```python
from build123d import *

# Parameters (mm, degrees)
SKETCH1_W               = 1041.4
SKETCH1_H               = 785.8125
BOSS_EXTRUDE1_DEPTH     = 6.35
CUT_EXTRUDE5_DEPTH      = 1305.62851711
F_1_4_CLEARANCE_HOLE1_D = 7.14248
CUT_EXTRUDE6_DEPTH      = 1305.62851711
SKETCH13_W              = 57.15
SKETCH13_H              = 25.4
CUT_EXTRUDE7_DEPTH      = 1305.62851711
FILLET1_R               = 6.35
FILLET1_OF_MIRROR1_R    = 6.35
CUT_EXTRUDE8_DEPTH      = 1305.62851711
LPATTERN1_COUNT         = 5
LPATTERN1_PITCH         = 222.25
CUT_EXTRUDE9_DEPTH      = 1305.62851711
LPATTERN2_COUNT         = 2
LPATTERN2_PITCH         = 457.2
FILLET2_R               = 6.35


with BuildPart() as part:
    # Sketch1 → Boss-Extrude1 (new body)
    with BuildSketch(Plane.XY):
        with Locations((520.7, 392.90625)):
            Rectangle(SKETCH1_W, SKETCH1_H)
    extrude(amount=BOSS_EXTRUDE1_DEPTH)

    # Sketch11 → Cut-Extrude5 (cut, through all)
    with BuildSketch(Plane.XY.offset(6.35)):
        with BuildLine():
            Line((346.3925, 640.207), (346.3925, 705.2945))
            ThreePointArc((346.3925, 705.2945), (343.2175, 708.4695), (346.3925, 711.6445))
            Line((346.3925, 711.6445), (354.0125, 711.6445))
            ThreePointArc((354.0125, 711.6445), (357.1875, 708.4695), (354.0125, 705.2945))
            Line((354.0125, 705.2945), (354.0125, 640.207))
            ThreePointArc((354.0125, 640.207), (357.1875, 637.032), (354.0125, 633.857))
            Line((354.0125, 633.857), (346.3925, 633.857))
            ThreePointArc((346.3925, 633.857), (343.2175, 637.032), (346.3925, 640.207))
        make_face()
        with BuildLine():
            Line((695.0075, 633.857), (687.3875, 633.857))
            ThreePointArc((687.3875, 633.857), (684.2125, 637.032), (687.3875, 640.207))
            Line((687.3875, 640.207), (687.3875, 705.2945))
            ThreePointArc((687.3875, 705.2945), (684.2125, 708.4695), (687.3875, 711.6445))
            Line((687.3875, 711.6445), (695.0075, 711.6445))
            ThreePointArc((695.0075, 711.6445), (698.1825, 708.4695), (695.0075, 705.2945))
            Line((695.0075, 705.2945), (695.0075, 640.207))
            ThreePointArc((695.0075, 640.207), (698.1825, 637.032), (695.0075, 633.857))
        make_face()
    extrude(amount=-CUT_EXTRUDE5_DEPTH, mode=Mode.SUBTRACT)

    # 1/4 Clearance Hole1 (through all)
    with Locations(Plane.XY.offset(6.35)):
        with Locations((54.102, 709.6125), (54.102, 76.2), (54.102, 392.90625), (987.298, 76.2), (987.298, 392.90625), (987.425, 709.6125), (336.8675, 672.75075), (363.5375, 672.75075), (677.8625, 672.75075), (704.5325, 672.75075)):
            Hole(F_1_4_CLEARANCE_HOLE1_D / 2)

    # Sketch12 → Cut-Extrude6 (cut, through all)
    with BuildSketch(Plane.XY.offset(6.35)):
        with BuildLine():
            Line((289.2425, 655.28825), (289.2425, 690.21325))
            ThreePointArc((289.2425, 690.21325), (303.53, 704.50075), (317.8175, 690.21325))
            Line((317.8175, 690.21325), (317.8175, 655.28825))
            ThreePointArc((317.8175, 655.28825), (303.53, 641.00075), (289.2425, 655.28825))
        make_face()
        with BuildLine():
            Line((752.1575, 655.28825), (752.1575, 690.21325))
            ThreePointArc((752.1575, 690.21325), (737.87, 704.50075), (723.5825, 690.21325))
            Line((723.5825, 690.21325), (723.5825, 655.28825))
            ThreePointArc((723.5825, 655.28825), (737.87, 641.00075), (752.1575, 655.28825))
        make_face()
    extrude(amount=-CUT_EXTRUDE6_DEPTH, mode=Mode.SUBTRACT)

    # Sketch13 → Cut-Extrude7 (cut, through all)
    with BuildSketch(Plane(origin=(0, 0, 0), x_dir=(-1, 0, 0), z_dir=(0, 0, -1))):
        with Locations((-1012.825, 627.0625)):
            Rectangle(SKETCH13_W, SKETCH13_H)
        with Locations((-1012.825, 291.7825)):
            Rectangle(SKETCH13_W, SKETCH13_H)
    cut_extrude7 = extrude(amount=-CUT_EXTRUDE7_DEPTH, mode=Mode.SUBTRACT)

    # Fillet1
    fillet1_edges = [part.edges().sort_by_distance(p)[0] for p in [
        (984.25, 639.7625, 3.175),
        (984.25, 614.3625, 3.175),
        (984.25, 304.4825, 3.175),
        (984.25, 279.0825, 3.175),
    ]]
    fillet(fillet1_edges, radius=FILLET1_R)

    # Mirror1: Cut-Extrude7 across plane
    add(cut_extrude7.mirror(Plane(origin=(520.7, 0, 0), x_dir=(0, 0, 1), z_dir=(1, 0, 0))), mode=Mode.SUBTRACT)

    # Fillet1 of Mirror1
    fillet1_of_mirror1_edges = [part.edges().sort_by_distance(p)[0] for p in [
        (57.15, 639.7625, 3.175),
        (57.15, 614.3625, 3.175),
        (57.15, 304.4825, 3.175),
        (57.15, 279.0825, 3.175),
    ]]
    fillet(fillet1_of_mirror1_edges, radius=FILLET1_OF_MIRROR1_R)

    # Sketch16 → Cut-Extrude8 (cut, through all)
    with BuildSketch(Plane.XY.offset(6.35)):
        with BuildLine():
            Line((66.675, 0), (85.725, 0))
            Line((85.725, 0), (85.725, 6.35))
            ThreePointArc((85.725, 6.35), (83.865128061, 10.840128061), (79.375, 12.7))
            Line((79.375, 12.7), (73.025, 12.7))
            ThreePointArc((73.025, 12.7), (68.534871939, 10.840128061), (66.675, 6.35))
            Line((66.675, 6.35), (66.675, 0))
        make_face()
    cut_extrude8 = extrude(amount=-CUT_EXTRUDE8_DEPTH, mode=Mode.SUBTRACT)

    # LPattern1: Cut-Extrude8 ×5
    with Locations(*[(i * LPATTERN1_PITCH, 0, 0) for i in range(1, LPATTERN1_COUNT)]):
        add(cut_extrude8, mode=Mode.SUBTRACT)

    # Sketch17 → Cut-Extrude9 (cut, through all)
    with BuildSketch(Plane.XY.offset(6.35)):
        with BuildLine():
            Line((419.1, 76.2), (165.1, 76.2))
            ThreePointArc((165.1, 76.2), (139.7, 101.6), (165.1, 127))
            Line((165.1, 127), (419.1, 127))
            ThreePointArc((419.1, 127), (444.5, 101.6), (419.1, 76.2))
        make_face()
    cut_extrude9 = extrude(amount=-CUT_EXTRUDE9_DEPTH, mode=Mode.SUBTRACT)

    # LPattern2: Cut-Extrude9 ×2
    with Locations(*[(i * LPATTERN2_PITCH, 0, 0) for i in range(1, LPATTERN2_COUNT)]):
        add(cut_extrude9, mode=Mode.SUBTRACT)

    # Fillet2
    fillet2_edges = [part.edges().sort_by_distance(p)[0] for p in [
        (0, 785.8125, 3.175),
        (0, 639.7625, 3.175),
        (0, 614.3625, 3.175),
        (0, 304.4825, 3.175),
        (0, 279.0825, 3.175),
        (0, 0, 3.175),
        (66.675, 0, 3.175),
        (85.725, 0, 3.175),
        (288.925, 0, 3.175),
        (307.975, 0, 3.175),
        (511.175, 0, 3.175),
        (530.225, 0, 3.175),
        (733.425, 0, 3.175),
        (752.475, 0, 3.175),
        (955.675, 0, 3.175),
        (974.725, 0, 3.175),
        (1041.4, 0, 3.175),
        (1041.4, 279.0825, 3.175),
        (1041.4, 304.4825, 3.175),
        (1041.4, 614.3625, 3.175),
        (1041.4, 639.7625, 3.175),
        (1041.4, 785.8125, 3.175),
    ]]
    fillet(fillet2_edges, radius=FILLET2_R - 0.0001)  # a hair under: the kernel refuses the full size


solid = part.part
```
Verification items for the finished model (mm, model axes). A direction names the side the tool comes from. Coordinates: 2 decimals unless noted, no trailing zeros. Loops run counter-clockwise (first coordinate to the right, second up) from the corner with the lowest first, then second, coordinate; pieces in that order, holes last. Notation, with made-up numbers: (70, 22) - (105, 22) arc R20 cw to (105, 59) - close; hole circle Ø3 at (62, 46). An arc over 180 degrees is marked (long way). Put each result on its own line as item: value.
Item 1: Set-up check for faces 1 (the face through (513, 398, 0)), 2 (the face through (901.694, 102.159, 3.219)): record each of +Z, -Z, +X, -X, +Y, -Y from which the full face is reachable in a straight line by a thin tool's end or side.
Conclusion:
face 1: -Z, +X, -X, +Y, -Y
face 2: +Z, -Z
Item 2: Gauge pin test, flat end, axial feed: pin 1 Ø9.5 at (x, y) = (677.86, 672.75) entering from +Z. Record the tip position at first contact, or that the pin passes through.
Conclusion:
pin 1: stops at z = 6.35
Item 3: Draft check along Y on faces 3 (the face through (444.494, 102.159, 3.219)), 4 (the face through (513, 398, 6.35)). Enter one of: pulls with the +Y half, pulls with the -Y half, needs draft (parallel to the pull), parting line crosses it, or undercut.
Conclusion:
face 3: undercut
face 4: needs draft
Item 4: Scan lines: line 1 along X through (y, z) = (393, 3); line 2 along Y through (x, z) = (231, 3); line 3 along X through (y, z) = (669, 3.5). Record each from-to range of solid material in increasing order.
Conclusion:
line 1: x = 0 to 50.53, 57.67 to 983.73, 990.87 to 1041.4
line 2: y = 0 to 76.2, 127 to 785.81
line 3: x = 0 to 289.24, 317.82 to 346.39, 354.01 to 687.39, 695.01 to 723.58, 752.16 to 1041.4
Item 5: Section check B-B (z = 1.5). Give the number of separate pieces and of enclosed holes in the cut face, then the cut area to 3 significant figures.
Conclusion:
separate pieces: 1
enclosed holes: 16
area: 776,000 mm2
Item 6: Section check A-A (x = 188.5). Enter the section's corners in (y, z), then the cut area to 3 significant figures.
Conclusion:
outline: (0, 0) - (76.2, 0) - (76.2, 6.35) - (0, 6.35) - close; (127, 0) - (785.81, 0) - (785.81, 6.35) - (127, 6.35) - close
area: 4,670 mm2
